For this review, take the finished solid that the model builds, in its own axes (mm). Face numbers are marked on the shaded views. A direction names the side the tool comes from. Coordinates: 2 decimals unless noted, no trailing zeros. Write each loop counter-clockwise with the first axis right and the second up, starting at its lowest first coordinate (ties: lowest second). Pieces come first, ordered by that corner, then holes. Notation, with made-up numbers: M -0.5,75.25 L 27.5,75.25 A21 ccw 27.5,111.25 Z; hole C 46.5,-15 d10. An arc over 180 degrees is marked long. Return JSON: item names as keys, results as strings.
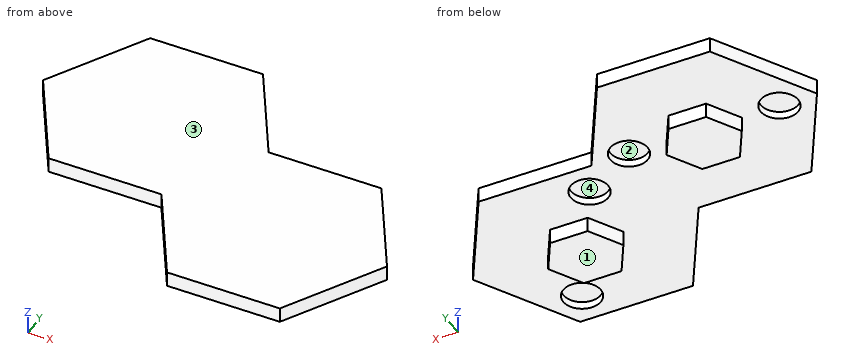
```python
from build123d import *

# Parameters (mm, degrees)
SKETCH1_R           = 5
BOSS_EXTRUDE1_DEPTH = 4
BOSS_EXTRUDE2_DEPTH = 8
SKETCH1_5_R         = 5
BOSS_EXTRUDE3_DEPTH = 2


with BuildPart() as part:
    # Sketch1 → Boss-Extrude1 (new body)
    with BuildSketch(Plane.XY):
        Polygon((-15, 25.980762114), (-30, 0), (-15, -25.980762114), (15, -25.980762114), (30, 0), (15, 25.980762114), align=None)
        with Locations((-20, 0)):
            Circle(SKETCH1_R, mode=Mode.SUBTRACT)
        with Locations((20, 0)):
            Circle(SKETCH1_R, mode=Mode.SUBTRACT)
        Polygon((-10, 0), (-5, -8.660254038), (5, -8.660254038), (10, 0), (5, 8.660254038), (-5, 8.660254038), align=None, mode=Mode.SUBTRACT)
    extrude(amount=-BOSS_EXTRUDE1_DEPTH)

    # Sketch1_4 → Boss-Extrude2 (add)
    with BuildSketch(Plane.XY):
        Polygon((-5, 8.660254038), (-10, 0), (-5, -8.660254038), (5, -8.660254038), (10, 0), (5, 8.660254038), align=None)
    extrude(amount=-BOSS_EXTRUDE2_DEPTH)

    # Sketch1_5 → Boss-Extrude3 (add)
    with BuildSketch(Plane.XY):
        with Locations((-20, 0)):
            Circle(SKETCH1_5_R)
        with Locations((20, 0)):
            Circle(SKETCH1_5_R)
    extrude(amount=-BOSS_EXTRUDE3_DEPTH)

    # Mirror1: part across plane


with BuildPart() as part_1:
    add(part.part)
    add(part.part.mirror(Plane(origin=(22.5, -12.990381057, -4), x_dir=(0, 0, 1), z_dir=(0.866025404, -0.5, 0))))


solid = part_1.part
```
1. We need section B-B (x = -20). State the section outline as (y, z) points.
Checks:
{"outline": "M -17.32,-4 L -5,-4 L -5,-2 L 5,-2 L 5,-4 L 17.32,-4 L 17.32,0 L -17.32,0 Z"}
2. We need section D-D (y = -7). State the section outline as (x, z) points.
Checks:
{"outline": "M -25.96,-4 L -5.96,-4 L -5.96,-8 L 5.96,-8 L 5.96,-4 L 30.28,-4 L 30.28,-2 L 39.72,-2 L 39.72,-4 L 64.04,-4 L 64.04,0 L -25.96,0 Z"}
3. We need section A-A (z = -6.25). State the section outline as (x, y) points.
Checks:
{"outline": "M -10,0 L -5,-8.66 L 5,-8.66 L 10,0 L 5,8.66 L -5,8.66 Z; M 35,-25.98 L 40,-34.64 L 50,-34.64 L 55,-25.98 L 50,-17.32 L 40,-17.32 Z"}
4. Clearance check with flat-ended pins moving along their axes: pin 1 Ø11 at (x, y) = (33, -10) entering from -Z; pin 2 Ø2 at (x, z) = (1, -6.5) entering from +Y; pin 3 Ø1.5 at (y, z) = (5.5, -1) entering from -X. State where each tip first meets the part, or that it passes through.
Checks:
{"pin 1": "z = -4", "pin 2": "y = 8.66", "pin 3": "x = -27.26"}
5. We need section C-C (y = -28.5). State the section outline as (x, z) points, plus the area to 3 significant figures.
Checks:
{"outline": "M 16.45,-4 L 36.45,-4 L 36.45,-8 L 53.55,-8 L 53.55,-4 L 73.55,-4 L 73.55,0 L 16.45,0 Z", "area": "297 mm2"}
6. Draft analysis for pull direction Y (two halves, no side actions). For the marked faces 1 and 2, state which applies: +Y half, -Y half, draft (parallel to the pull), parting line (faces both ways), or undercut.
Checks:
{"face 1": "draft", "face 2": "undercut"}
7. Wall thickness on L1, parallel to Y at x = 35, z = -3.3; L2, parallel to Y at x = 55, z = -3.1; L3, parallel to Z at x = 54.5, y = -36: over which ranges is each line inside the solid? List them lowest first. Write a range as from..to.
Checks:
{"L1": "-51.96..-13.66, -3.66..0", "L2": "-51.96..-48.3, -38.3..0", "L3": "-4..0"}
8. For the marked faces 3 and 4, list the 3-axis set-ups (+Z, -Z, +X, -X, +Y, -Y) from which the entire face can be reached by the end or side of a thin tool; tool diameter is ignored.
Checks:
{"face 3": "+Z, +X, -X, +Y, -Y", "face 4": "-Z"}
